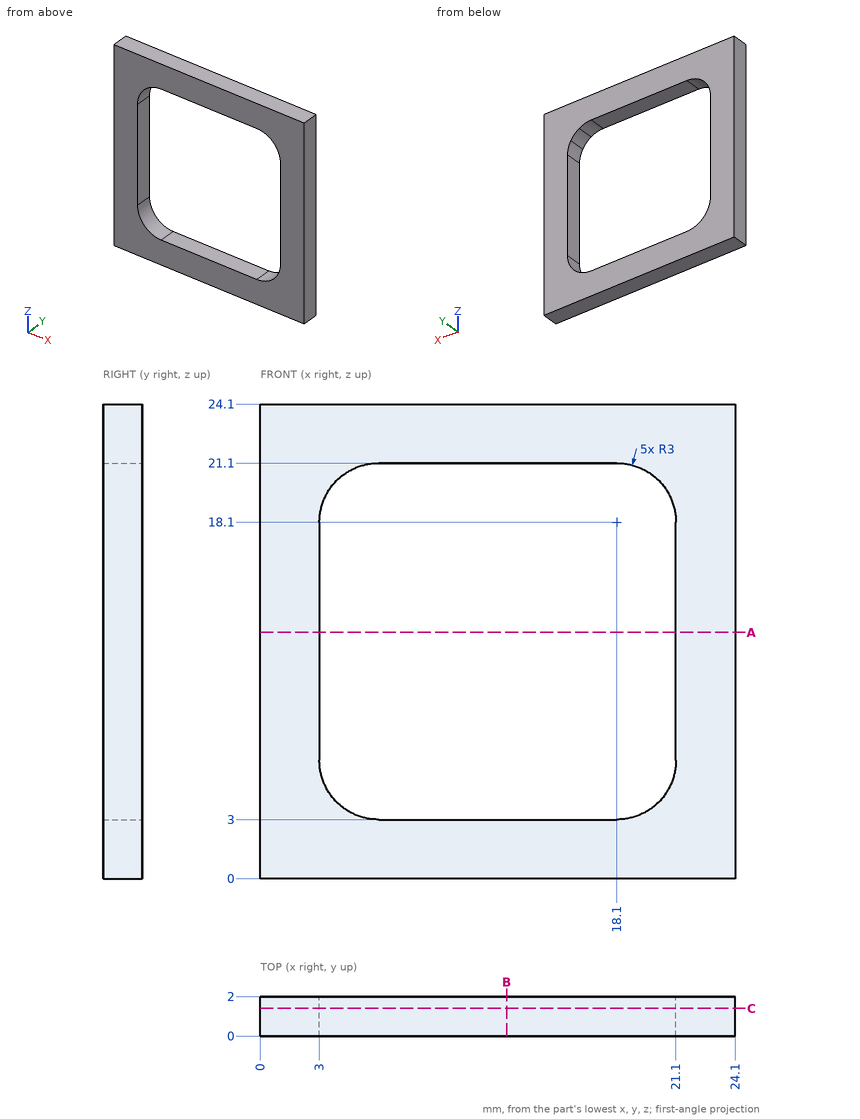
Source: three-view drawing plus pictorial views. Frame: mm from the lowest corner of the part. Round coordinates to 2 decimals unless told otherwise and drop trailing zeros. Loops run counter-clockwise (first coordinate to the right, second up) from the corner with the lowest first, then second, coordinate; pieces in that order, holes last.
Q1. Section B-B on x = 12.5. Return loops of the section in (y, z), plus the area to 3 significant figures.
Q2. Material intervals for L1, parallel to X at y = 0.5, z = 12; L2, parallel to Z at x = 19, y = 1.65, sorted ascending.
Q3. Section A-A on z = 12.5. Return loops of the section in (x, y).
Q4. Pin query (flat end, axial travel): P1, Ø1, axis at x = 9.5, y = 1, coming from the -Z side. Return the tip coordinate at first contact, or that it passes through.
Q5. Section C-C on y = 1.4. Return loops of the section in (x, z).
Evaluation:
1. outline: (0, 0) - (2, 0) - (2, 3) - (0, 3) - close; (0, 21.1) - (2, 21.1) - (2, 24.1) - (0, 24.1) - close
1. area: 12.0 mm2
2. L1: x = 0 to 3, 21.1 to 24.1
2. L2: z = 0 to 3.14, 20.96 to 24.1
3. outline: (0, 0) - (3, 0) - (3, 2) - (0, 2) - close; (21.1, 0) - (24.1, 0) - (24.1, 2) - (21.1, 2) - close
4. P1: stops at z = 0
5. outline: (0, 0) - (24.1, 0) - (24.1, 24.1) - (0, 24.1) - close; hole (3, 6) arc R3 ccw to (6, 3) - (18.1, 3) arc R3 ccw to (21.1, 6) - (21.1, 18.1) arc R3 ccw to (20.68, 19.62) arc R3 ccw to (19.62, 20.68) arc R3 ccw to (18.1, 21.1) - (6, 21.1) arc R3 ccw to (3, 18.1) - close
